Here's how the part is built. I have some questions about the finished solid (model axes, mm). A direction names the side the tool comes from. Coordinates: 2 decimals unless noted, no trailing zeros. Loops run counter-clockwise (first coordinate to the right, second up) from the corner with the lowest first, then second, coordinate; pieces in that order, holes last. Notation, with made-up numbers: (77.5, 52) -> (95.5, 52) arc R15 ccw to (95.5, 67) -> close; hole circle Ø3 at (20.5, -33.5). An arc over 180 degrees is marked (long way). Answer as a JSON object with one key per item and string values. Group by question number.
Q1. On a 3-axis mill with a long thin cutter (end or side, diameter ignored), from which of +Z, -Z, +X, -X, +Y, -Y can I reach the whole of each face in a straight line? I mean faces 4 (the cylindrical face through (0.42, -27.27, 167.2)), 5 (the cylindrical face through (-28.496, -48.688, 179.342)), 6 (the flat face through (-0.84, 11.59, 138.87)), 7 (the flat face through (0.91, 111.75, 130.92)), 8 (the cylindrical face through (68.574, 113.036, 131.73)). Say none if no direction works.
Q2. I want a section at B-B on y = -15.5. Write out the boundary of the cut face in (x, z).
Q3. I'm going to push flat-ended pins straight in: pin 1 (7.5 mm diameter, centred on x = 66, z = 181, fed in from -Y); pin 2 (24.5 mm diameter, centred on y = -23.5, z = 187.5, fed in from +X). Where does each tip first touch, or does it pass through?
Q4. Thinking about a two-plate mould opening in Y: for faces 1 (the flat face through (1, 69, 200)), 2 (the flat face through (63, 143.846, 180)), 3 (the flat face through (0, -70, 196)), which applies, released by +Y, released by -Y, zero draft, split by the parting line, or undercut?
Q5. I want a section at A-A on x = -19. Write out the boundary of the cut face in (y, z).
Q6. I need wall thicknesses on line 1 (Z direction, x = -1, y = 141); line 2 (X direction, y = -31, z = 186.5); line 3 (Y direction, x = 4.5, z = 121.5). Which ranges of each line are inside material? Lowest first, please.
Autodesk Fusion 360 part; units mm, degrees
sketch "Boceto1" plane through (0, 0, 0) normal (0, 1, 0) x (1, 0, 0)
  line L0 (0, -200) -> (70, -200)
  line L1 (0, -200) -> (-70, -200)
  line L2 (-70, -200) -> (-70, 0)
  line L3 (-70, 0) -> (70, 0)
  line L4 (70, 0) -> (70, -200)
  dimension "d1" = 200
  dimension "d2" = 70
  dimension "d3" = 70
extrude "Extruir1" add sketch "Boceto1" along normal blind 160
sketch "Boceto2" plane through (70, 0, 0) normal (1, 0, 0) x (0, 1, 0)
  line L0 (0, 200) -> (0, 0)
  line L1 (0, 0) -> (160, 0)
  line L2 (160, 0) -> (160, 200)
  line L3 (160, 200) -> (0, 200)
  line L4 (140, 0) -> (0, 140)
  line L5 (430, 170) -> (420, 170)
extrude "Extruir2" cut sketch "Boceto2" against normal blind 140 contours L0 L1 L4
sketch "Boceto3" plane through (0, 0, 0) normal (0, -1, 0) x (1, 0, 0)
  line L0 (-70, 140) -> (70, 140)
  line L1 (70, 140) -> (70, 200)
  line L2 (70, 200) -> (-70, 200)
  line L3 (-70, 200) -> (-70, 140)
  line L4 (30, 200) -> (30, 190)
  line L5 (30, 190) -> (-30, 190)
  line L6 (-30, 190) -> (-30, 200)
extrude "Extruir3" add sketch "Boceto3" along normal blind 70 contours L2 L4 L5 L6
sketch "Boceto4" plane through (0, 0, 190) normal (0, 0, -1) x (1, 0, 0)
  line L0 (-30, 0) -> (30, 0)
  line L1 (30, 0) -> (30, 70)
  line L2 (30, 70) -> (-30, 70)
  line L3 (-30, 70) -> (-30, 0)
  line L4 (-30, 20) -> (30, 20)
revolve "Revolución1" add sketch "Boceto4" angle 30 about axis through (30, -70, 190) along (-1, 0, 0) contours L1 L2 L3 L4
sketch "Boceto5" plane through (0, 64.7724, 112.1891) normal (0, -0.5, -0.866) x (1, 0, 0)
  line L0 (-30, 105.6218) -> (30, 105.6218)
  line L1 (30, 105.6218) -> (30, 155.6218)
  line L2 (30, 155.6218) -> (-30, 155.6218)
  line L3 (-30, 155.6218) -> (-30, 105.6218)
  circle A0 centre (-15, 130) radius 10
  circle A1 centre (-15, 130) radius 7.5
  dimension "d11" = 15
extrude "Extruir4" cut sketch "Boceto5" against normal blind 5 contours A1
sketch "Boceto6" plane through (0, 64.7724, 112.1891) normal (0, -0.5, -0.866) x (1, 0, 0)
  circle A0 centre (-15, 130) radius 7.5
  line L0 (-30, 105.6218) -> (30, 105.6218)
  line L1 (30, 105.6218) -> (30, 155.6218)
  line L2 (30, 155.6218) -> (-30, 155.6218)
  line L3 (-30, 155.6218) -> (-30, 105.6218)
  circle A1 centre (-15, 130) radius 10
  dimension "d14" = 20
sketch "Boceto7" plane through (70, 0, 0) normal (1, 0, 0) x (0, 1, 0)
  line L0 (0, 140) -> (140, 0)
  line L1 (140, 0) -> (160, 0)
  line L2 (160, 0) -> (160, 200)
  line L3 (160, 200) -> (0, 200)
  line L4 (0, 200) -> (0, 140)
  line L5 (0, 140) -> (0, 160)
  line L6 (0, 160) -> (160, 0)
  circle A0 centre (130, 80) radius 20
  circle A1 centre (60, 160) radius 20
  line L7 (45.8852, 145.8306) -> (114.9426, 66.8366)
  line L8 (147.3803, 89.8957) -> (75.0996, 173.1149)
  dimension "d15" = 20
extrude "Extruir5" cut sketch "Boceto7" against normal blind 170 contours A0 L8 | A0 A1 L7 L8 | A1 picked at (118.5803, 82.9284)
sketch "Boceto8" plane through (0, 70, 70) normal (0, -0.7071, -0.7071) x (1, 0, 0)
  line L0 (70, -98.9949) -> (70, 98.9949)
  line L1 (70, 98.9949) -> (-70, 98.9949)
  line L2 (-70, 98.9949) -> (-70, -98.9949)
  line L3 (-70, -98.9949) -> (70, -98.9949)
  line L4 (-60, 90) -> (60, 90)
  line L5 (60, 90) -> (60, -90)
  line L6 (-60, 90) -> (-60, -90)
  line L7 (-60, -90) -> (60, -90)
extrude "Extruir6" cut sketch "Boceto8" against normal blind 15 contours L4 L5 L6 L7
sketch "Boceto9" plane through (70, 0, 0) normal (1, 0, 0) x (0, 1, 0)
  arc A0 (75.0996, 173.1149) -> (45.8852, 145.8306) centre (60, 160) ccw
  line L0 (75.0996, 173.1149) -> (147.3803, 89.8957)
  arc A1 (114.9426, 66.8366) -> (147.3803, 89.8957) centre (130, 80) ccw
  line L1 (114.9426, 66.8366) -> (45.8852, 145.8306)
  line L2 (0, 140) -> (140, 0)
  line L3 (140, 0) -> (160, 0)
  line L4 (160, 0) -> (160, 200)
  line L5 (160, 200) -> (0, 200)
  line L6 (0, 200) -> (0, 140)
  line L7 (140, 190) -> (150, 190)
  line L8 (150, 190) -> (150, 170)
  line L9 (150, 170) -> (140, 170)
  line L10 (147, 171) -> (147, 189)
  line L11 (147, 189) -> (149, 189)
  line L12 (149, 189) -> (149, 171)
  line L13 (149, 171) -> (147, 171)
  line L14 (143.8463, 170) -> (143.8463, 190)
  dimension "d20" = 20
extrude "Extruir7" cut sketch "Boceto9" against normal blind 15 contours L7 L8 L9 L14
fillet "Empalme1" radius 5 19 edges at (70, 0, 170) (70, 70, 70) (70, 150, 0) (70, 160, 100) (-70, 0, 170) (-70, 70, 70) (-70, 150, 0) (-70, 160, 100) (-70, 80.4139, 106.3336) (-70, 141.5879, 63.6991) (-70, 111.24, 131.5053) (-70, 46.349, 174.6167) (70, 141.5879, 63.6991) (70, 80.4139, 106.3336) (70, 46.349, 174.6167) (70, 111.24, 131.5053) (0, 160, 0) (0, 140, 0) (0, 0, 140)
fillet "Empalme2" radius 5 4 edges at (30, -48.3494, 177.5) (0, -26.6987, 165) (-30, -48.3494, 177.5) (0, -70, 190)
Result set:
{
 "1": {"face 4": "-Z, +X, -X", "face 5": "-Z, -X, -Y", "face 6": "-Z", "face 7": "+X, -X", "face 8": "+X"},
 "2": {"outline": "(-30, 190) -> (30, 190) -> (30, 200) -> (-30, 200) -> close"},
 "3": {"pin 1": "stops at y = 0", "pin 2": "stops at x = 30"},
 "4": {"face 1": "zero draft", "face 2": "undercut", "face 3": "released by -Y"},
 "5": {"outline": "(-70, 192.89) arc R5 ccw to (-67.5, 188.56) -> (-53.31, 180.36) -> (-50.81, 184.69) -> (-39.82, 178.35) -> (-42.32, 174.02) -> (-31.27, 167.64) arc R5 ccw to (-24.19, 169.97) arc R50 ccw to (-20, 190) -> (0, 190) -> (0, 142.07) arc R5 ccw to (1.46, 138.54) -> (6.36, 133.64) -> (16.97, 144.25) -> (144.25, 16.97) -> (133.64, 6.36) -> (138.54, 1.46) arc R5 ccw to (142.07, 0) -> (155, 0) arc R5 ccw to (160, 5) -> (160, 200) -> (-70, 200) -> close; hole (45.89, 145.83) -> (114.94, 66.84) arc R20 ccw to (147.38, 89.9) -> (75.1, 173.11) arc R20 ccw (long way) to start"},
 "6": {"line 1": "z = 0.12 to 13.72, 20.21 to 63.3, 97.24 to 200", "line 2": "x = -30 to 30", "line 3": "y = 39.71 to 67.16, 119.93 to 160"}
}
